```python
from build123d import *

# Parameters (mm, degrees)
SKETCH1_W           = 87
SKETCH1_H           = 60
BOSS_EXTRUDE1_DEPTH = 65
SKETCH2_W           = 83
SKETCH2_H           = 56
CUT_EXTRUDE1_DEPTH  = 62
SKETCH3_W           = 18
SKETCH3_H           = 15
CUT_EXTRUDE2_DEPTH  = 57
SKETCH4_R           = 6
CUT_EXTRUDE3_DEPTH  = 24
SKETCH5_W           = 34
SKETCH5_H           = 30
CUT_EXTRUDE4_DEPTH  = 24
CUT_EXTRUDE5_DEPTH  = 117
SKETCH7_W           = 73
SKETCH7_H           = 46
CUT_EXTRUDE6_DEPTH  = 10


with BuildPart() as part:
    # Sketch1 → Boss-Extrude1 (new body)
    with BuildSketch(Plane(origin=(0, 0, 0), x_dir=(1, 0, 0), z_dir=(0, 1, 0))):
        with Locations((-43.5, 30)):
            Rectangle(SKETCH1_W, SKETCH1_H)
    extrude(amount=BOSS_EXTRUDE1_DEPTH)

    # Sketch2 → Cut-Extrude1 (cut)
    with BuildSketch(Plane(origin=(0, 65, 0), x_dir=(1, 0, 0), z_dir=(0, 1, 0))):
        with Locations((-43.5, 30)):
            Rectangle(SKETCH2_W, SKETCH2_H)
    extrude(amount=-CUT_EXTRUDE1_DEPTH, mode=Mode.SUBTRACT)

    # Sketch3 → Cut-Extrude2 (cut)
    with BuildSketch(Plane(origin=(0, 0, 0), x_dir=(0, 0, -1), z_dir=(1, 0, 0))):
        with Locations((30, 17.5)):
            Rectangle(SKETCH3_W, SKETCH3_H)
    extrude(amount=-CUT_EXTRUDE2_DEPTH, mode=Mode.SUBTRACT)

    # Sketch4 → Cut-Extrude3 (cut)
    with BuildSketch(Plane.XY):
        with Locations((-60, 25)):
            Circle(SKETCH4_R)
    extrude(amount=-CUT_EXTRUDE3_DEPTH, mode=Mode.SUBTRACT)

    # Sketch5 → Cut-Extrude4 (cut)
    with BuildSketch(Plane.ZY.offset(87)):
        with Locations((-30, 25)):
            Rectangle(SKETCH5_W, SKETCH5_H)
    extrude(amount=-CUT_EXTRUDE4_DEPTH, mode=Mode.SUBTRACT)

    # Sketch6 → Cut-Extrude5 (cut)
    with BuildSketch(Plane(origin=(0, 0, 0), x_dir=(0, 0, -1), z_dir=(1, 0, 0))):
        Polygon((8.464101615, 65), (5, 59), (55, 59), (51.535898385, 65), align=None)
    extrude(amount=-CUT_EXTRUDE5_DEPTH, mode=Mode.SUBTRACT)

    # Sketch7 → Cut-Extrude6 (cut)
    with BuildSketch(Plane(origin=(0, 3, 0), x_dir=(1, 0, 0), z_dir=(0, 1, 0))):
        with Locations((-43.5, 30)):
            Rectangle(SKETCH7_W, SKETCH7_H)
    extrude(amount=-CUT_EXTRUDE6_DEPTH, mode=Mode.SUBTRACT)


solid = part.part
```
Verification items for the finished model (mm, model axes). A direction names the side the tool comes from. Give positions to 0.01 mm unless a question says otherwise; leave off trailing zeros. Order: outer loops, then holes, each group sorted by start corner. A loop starts at its lowest first (then second) coordinate and runs counter-clockwise, first axis right, second up. Notation, with made-up numbers: (-21.75, -20.5) - (-11.75, -20.5) arc R22 cw to (-11.75, -10.5) - close; hole circle Ø3 at (35.25, 30.5). An arc over 180 degrees is marked (long way). Answer as CSV lines item,"result". Start each with the question number.
Item 1: Mould release check, pull along Z, two halves, no side actions. Record for faces 5 (the face through (-44, 65, -59)), 6 (the face through (-85.99, 61.96, -53.29)), 7 (the face through (-44, 32, -60)): released by +Z, released by -Z, zero draft, split by the parting line, or undercut.
Item 2: Section check A-A, the plane x = -60. Record the boundary of the cut face in (y, z), plus the area to 3 significant figures.
Item 3: Section check B-B, the plane z = -17. Record the boundary of the cut face in (x, y), plus the area to 3 significant figures.
Item 4: Material ranges on L1, parallel to Z at x = -72, y = 17; L2, parallel to Y at x = -60, z = -1.45; L3, parallel to X at y = 62, z = -3, recorded low to high.
Item 5: Section check C-C, the plane y = 54. Record the boundary of the cut face in (x, z).
Item 6: Access from +Z, -Z, +X, -X, +Y, -Y to the whole of each face (thin tool, end or side, straight path). Record for faces 1 (the face through (-85, 41, -30)), 2 (the face through (-86, 25, -47)), 3 (the face through (-7, 2, -30)), 4 (the face through (-0.986, 62.042, -6.756)).
Item 7: Section check D-D, the plane x = -48. Record the boundary of the cut face in (y, z), plus the area to 3 significant figures.
Item 8: Gauge pin test, flat ends, axial feed: pin 1 (1 mm diameter, centred on x = -1.5, z = -26.5, fed in from +Y); pin 2 (10 mm diameter, centred on y = 34, z = -34.5, fed in from -X). Record the tip position at first contact, or that the pin passes through.
Filled in:
1,face 5,"zero draft"
1,face 6,"undercut"
1,face 7,"released by -Z"
2,outline,"(0, -60) - (65, -60) - (65, -58) - (3, -58) - (3, -53) - (0, -53) - close; (0, -7) - (3, -7) - (3, -2) - (19, -2) - (19, 0) - (0, 0) - close; (31, -2) - (65, -2) - (65, 0) - (31, 0) - close"
2,area,"266 mm^2"
3,outline,"(-87, 0) - (-80, 0) - (-80, 3) - (-85, 3) - (-85, 10) - (-87, 10) - close; (-87, 40) - (-85, 40) - (-85, 59) - (-87, 59) - close; (-7, 0) - (0, 0) - (0, 59) - (-2, 59) - (-2, 3) - (-7, 3) - close"
3,area,"206 mm^2"
4,L1,"-60 to -58, -2 to 0"
4,L2,"0 to 19, 31 to 65"
4,L3,"-87 to -85, -2 to 0"
5,outline,"(-87, -60) - (0, -60) - (0, 0) - (-87, 0) - close; hole (-85, -58) - (-2, -58) - (-2, -2) - (-85, -2) - close"
6,face 1,"+Y"
6,face 2,"-X"
6,face 3,"+Y, -Y"
6,face 4,"+X, -X"
7,outline,"(0, -60) - (65, -60) - (65, -58) - (3, -58) - (3, -53) - (0, -53) - close; (0, -7) - (3, -7) - (3, -2) - (65, -2) - (65, 0) - (0, 0) - close"
7,area,"290 mm^2"
8,pin 1,"y = 59"
8,pin 2,"x = -2"
